```python
from build123d import *

# Parameters (mm, degrees)
SKETCH_1_W      = 40
SKETCH_1_H      = 20
EXTRUDE_1_DEPTH = 26.9
SKETCH_2_R      = 1.863789346
EXTRUDE_2_DEPTH = 2.6
SKETCH_3_W      = 40
SKETCH_3_H      = 20
EXTRUDE_3_DEPTH = 8
SKETCH_4_R      = 4
EXTRUDE_4_DEPTH = 6
SKETCH_5_R      = 10.5
EXTRUDE_5_DEPTH = 2.2


with BuildPart() as part:
    # 草图1 → 凸台-拉伸1 (new body)
    with BuildSketch(Plane(origin=(0, 0, 0), x_dir=(1, 0, 0), z_dir=(0, 1, 0))):
        with Locations((-10, 0)):
            Rectangle(SKETCH_1_W, SKETCH_1_H)
    extrude(amount=-EXTRUDE_1_DEPTH)

    # 草图2 → 凸台-拉伸2 (add)
    with BuildSketch(Plane(origin=(0, 0, 0), x_dir=(1, 0, 0), z_dir=(0, 1, 0))):
        with BuildLine():
            Line((-35, -10), (15, -10))
            ThreePointArc((15, -10), (16.414213562, -9.414213562), (17, -8))
            Line((17, -8), (17, 8))
            ThreePointArc((17, 8), (16.414213562, 9.414213562), (15, 10))
            Line((15, 10), (-35, 10))
            ThreePointArc((-35, 10), (-36.414213562, 9.414213562), (-37, 8))
            Line((-37, 8), (-37, -8))
            ThreePointArc((-37, -8), (-36.414213562, -9.414213562), (-35, -10))
        make_face()
        with Locations(Location((-34.3, -4.95, 0), (0, 0, 270))):
            Circle(SKETCH_2_R, mode=Mode.SUBTRACT)
        with Locations(Location((-34.3, 4.95, 0), (0, 0, 270))):
            Circle(SKETCH_2_R, mode=Mode.SUBTRACT)
        with Locations(Location((14.3, -4.95, 0), (0, 0, 270))):
            Circle(SKETCH_2_R, mode=Mode.SUBTRACT)
        with Locations(Location((14.3, 4.95, 0), (0, 0, 270))):
            Circle(SKETCH_2_R, mode=Mode.SUBTRACT)
    extrude(amount=EXTRUDE_2_DEPTH)

    # 草图3 → 凸台-拉伸3 (add)
    with BuildSketch(Plane(origin=(0, 2.6, 0), x_dir=(1, 0, 0), z_dir=(0, 1, 0))):
        with Locations((-10, 0)):
            Rectangle(SKETCH_3_W, SKETCH_3_H)
    extrude(amount=EXTRUDE_3_DEPTH)

    # 草图4 → 凸台-拉伸4 (add)
    with BuildSketch(Plane(origin=(0, 10.6, 0), x_dir=(1, 0, 0), z_dir=(0, 1, 0))):
        with Locations(Location((0, 0, 0), (0, 0, 270))):
            Circle(SKETCH_4_R)
    extrude(amount=EXTRUDE_4_DEPTH)

    # 草图5 → 凸台-拉伸5 (add)
    with BuildSketch(Plane(origin=(0, 16.6, 0), x_dir=(1, 0, 0), z_dir=(0, 1, 0))):
        with Locations(Location((0, 0, 0), (0, 0, 270))):
            Circle(SKETCH_5_R)
    extrude(amount=EXTRUDE_5_DEPTH)


solid = part.part
```
Geometry: final body of the model. Coordinates: model frame, mm. A direction names the side the tool comes from. Round coordinates to 2 decimals unless told otherwise and drop trailing zeros. Loops run counter-clockwise (first coordinate to the right, second up) from the corner with the lowest first, then second, coordinate; pieces in that order, holes last. Notation, with made-up numbers: (-27, 60) -> (18, 60) arc R15 cw to (18, 83) -> close; hole circle Ø5 at (-31.75, 17.25). An arc over 180 degrees is marked (long way). Use one line per item in the form item = value. Start each with the question number.
1) First-contact query: P1, Ø3.5, axis at x = 14.5, z = -2.5, coming from the -Y side; P2, Ø5, axis at y = 8, z = -5, coming from the -X side; P3, Ø6, axis at x = -8.5, y = -9.5, coming from the -Z side. Flat tips, straight axial feed; report the tip coordinate or a pass-through.
2) Section D-D on z = 0. Output: boundary loops of the cut face in (x, y).
3) Line query: L1, parallel to X at y = 1.6, z = -4.95; L2, parallel to Y at x = -2.5, z = -8; L3, parallel to Z at x = -34, y = 1. Output: solid intervals per line, ascending.
4) Access query for faces 4 (the cylindrical face through (-3.905, 13.558, -0.867)), 5 (the cylindrical face through (3.2, 17.7, 10)), 6 (the flat face through (-30, -13, 0)). Directions: +Z, -Z, +X, -X, +Y, -Y. A direction counts if a zero-diameter tool reaches every point of the face in a straight line with its end or side. Return the directions, or none.
5) Section C-C on z = -5.25. Output: boundary loops of the cut face in (x, y), then the cut area to 3 significant figures.
6) Section B-B on y = 1. Output: boundary loops of the cut face in (x, z).
7) Section A-A on x = -34.3. Output: boundary loops of the cut face in (y, z).
8) Draft query along Y for faces 1 (the flat face through (-34, 0, 0)), 2 (the flat face through (-10, 10.6, 0)), 3 (the cylindrical face through (16.4, 1.28, 9.43)). Return one class per face: released by +Y, released by -Y, zero draft, split by the parting line, or undercut.
Response:
q1.P1 = 0
q1.P2 = -30
q1.P3 = -10
q2.outline = (-37, 0) -> (-30, 0) -> (-30, -26.9) -> (10, -26.9) -> (10, 0) -> (17, 0) -> (17, 2.6) -> (10, 2.6) -> (10, 10.6) -> (4, 10.6) -> (4, 16.6) -> (10.5, 16.6) -> (10.5, 18.8) -> (-10.5, 18.8) -> (-10.5, 16.6) -> (-4, 16.6) -> (-4, 10.6) -> (-30, 10.6) -> (-30, 2.6) -> (-37, 2.6) -> close
q3.L1 = -37 to -36.16, -32.44 to 12.44, 16.16 to 17
q3.L2 = -26.9 to 10.6, 16.6 to 18.8
q3.L3 = -10 to -6.79, -3.11 to 3.11, 6.79 to 10
q4.face_4 = none
q4.face_5 = +Y
q4.face_6 = +Z, -Z, -X, -Y
q5.outline = (-37, 0) -> (-36.14, 0) -> (-36.14, 2.6) -> (-37, 2.6) -> close; (-32.46, 0) -> (-30, 0) -> (-30, -26.9) -> (10, -26.9) -> (10, 0) -> (12.46, 0) -> (12.46, 2.6) -> (10, 2.6) -> (10, 10.6) -> (-30, 10.6) -> (-30, 2.6) -> (-32.46, 2.6) -> close; (-9.09, 16.6) -> (9.09, 16.6) -> (9.09, 18.8) -> (-9.09, 18.8) -> close; (16.14, 0) -> (17, 0) -> (17, 2.6) -> (16.14, 2.6) -> close
q5.area = 1,560 mm^2
q6.outline = (-37, -8) arc R2 ccw to (-35, -10) -> (15, -10) arc R2 ccw to (17, -8) -> (17, 8) arc R2 ccw to (15, 10) -> (-35, 10) arc R2 ccw to (-37, 8) -> close; hole circle Ø3.73 at (-34.3, -4.95); hole circle Ø3.73 at (-34.3, 4.95); hole circle Ø3.73 at (14.3, -4.95); hole circle Ø3.73 at (14.3, 4.95)
q7.outline = (0, -10) -> (2.6, -10) -> (2.6, -6.81) -> (0, -6.81) -> close; (0, -3.09) -> (2.6, -3.09) -> (2.6, 3.09) -> (0, 3.09) -> close; (0, 6.81) -> (2.6, 6.81) -> (2.6, 10) -> (0, 10) -> close
q8.face_1 = released by -Y
q8.face_2 = undercut
q8.face_3 = zero draft
